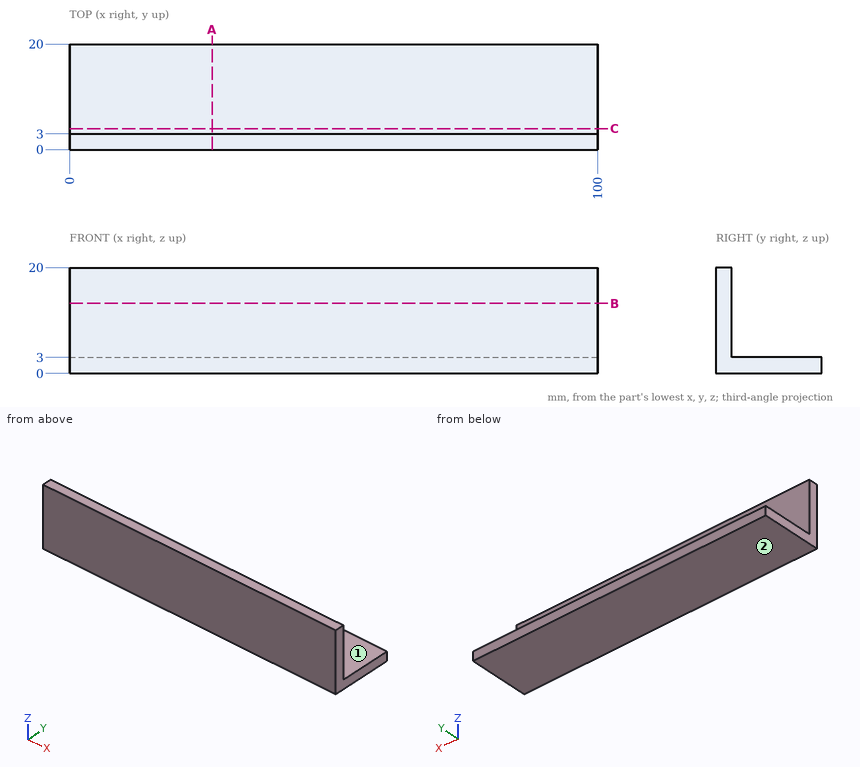
Verification items for this drawing (mm, ordinates from the low corner). A direction names the side the tool comes from. Give positions to 0.01 mm unless a question says otherwise; leave off trailing zeros. Write each loop counter-clockwise with the first axis right and the second up, starting at its lowest first coordinate (ties: lowest second). Pieces come first, ordered by that corner, then holes. Notation, with made-up numbers: (59.25, 17.5) -> (71.25, 17.5) arc R36 cw to (71.25, 56.5) -> close; hole circle Ø9 at (3, 32). An arc over 180 degrees is marked (long way). Use CSV: the item, a comma, the result in double quotes.
(1) Material ranges on L1, parallel to Z at x = 18, y = 6, recorded low to high.
Derived:
L1,"z = 0 to 3"
(2) Sectioned sample at B-B (z = 13.25). Record the cut outline in (x, y), plus the area to 3 significant figures.
Derived:
outline,"(0, 0) -> (100, 0) -> (100, 3) -> (0, 3) -> close"
area,"300 mm^2"
(3) Sectioned sample at A-A (x = 27). Record the cut outline in (y, z).
Derived:
outline,"(0, 0) -> (20, 0) -> (20, 3) -> (3, 3) -> (3, 20) -> (0, 20) -> close"
(4) Set-up check for the marked faces 1 and 2: record each of +Z, -Z, +X, -X, +Y, -Y from which the full face is reachable in a straight line by a thin tool's end or side.
Derived:
face 1,"+Z, +X, -X, +Y"
face 2,"-Z, +X, -X, +Y, -Y"
(5) Go/stop test with flat-tipped pins: pin 1 (5 mm diameter, centred on x = 32, z = 9, fed in from +Y); pin 2 (5 mm diameter, centred on x = 63.5, y = 15.5, fed in from +Z). Record where each tip stops, or that it passes through.
Derived:
pin 1,"stops at y = 3"
pin 2,"stops at z = 3"
